Can you work these out from the model? Positions are in its coordinate system, mm. Give positions to 0.01 mm unless a question says otherwise; leave off trailing zeros. Loops run counter-clockwise (first coordinate to the right, second up) from the corner with the lowest first, then second, coordinate; pieces in that order, holes last. Notation, with made-up numbers: (70, 36.5) - (111, 36.5) arc R12 ccw to (111, 47.5) - close; hole circle Ø8 at (74, 37). An arc over 180 degrees is marked (long way). Answer in a Markdown table with one row per item.
Autodesk Inventor part; units mm, degrees
ref_plane "YZ Plane" through (0, 0, 0) normal (1, 0, 0) x (0, 1, 0)
ref_plane "XZ Plane" through (0, 0, 0) normal (0, 1, 0) x (-1, 0, 0)
ref_plane "XY Plane" through (0, 0, 0) normal (0, 0, 1) x (1, 0, 0)
sketch "Sketch1" plane through (0, 0, 0) normal (0, 1, 0) x (-1, 0, 0)
  circle A0 centre (0, 0) radius 12.7
  dimension "d0" = 25.4
extrude "Extrusion1" add sketch "Sketch1" along normal blind 5.8674
sketch "Sketch2" plane through (0, 5.8674, 0) normal (0, 1, 0) x (1, 0, 0)
  line L0 (0, 0) -> (-7.7692, 0)
  line L1 (-7.7692, 0) -> (-7.7692, 6.975)
  line L2 (-7.7692, 6.975) -> (0, 6.975)
  line L3 (0, 6.975) -> (0, 0)
extrude "Extrusion2" cut sketch "Sketch2" against normal blind 254
sketch "Sketch3" plane through (0, 5.8674, 0) normal (0, 1, 0) x (1, 0, 0)
  line L0 (0, 6.018) -> (5.0945, 6.018)
  line L1 (5.0945, 6.018) -> (5.0945, 4.5769)
  line L2 (5.0945, 4.5769) -> (0, 4.5769)
  line L3 (0, 4.5769) -> (0, 6.018)
  point P0 (0, 0)
extrude "Extrusion3" cut sketch "Sketch3" against normal blind 254
sketch "Sketch4" plane through (0, 5.8674, 0) normal (0, 1, 0) x (1, 0, 0)
  circle A0 centre (-2.0297, 0) radius 3.9608
  point P0 (0, 0)
extrude "Extrusion4" cut sketch "Sketch4" against normal blind 254
sketch "Sketch5" plane through (0, 5.8674, 0) normal (0, 1, 0) x (1, 0, 0)
  line L0 (12.2968, 4.5116) -> (-14.5211, 4.5116)
  line L1 (-14.5211, 4.5116) -> (-14.5211, 13.7027)
  line L2 (-14.5211, 13.7027) -> (12.2968, 13.7027)
  line L3 (12.2968, 13.7027) -> (12.2968, 4.5116)
  point P0 (0, 0)
extrude "Extrusion5" cut sketch "Sketch5" against normal blind 254
sketch "Sketch6" plane through (0, 5.8674, 0) normal (0, 1, 0) x (1, 0, 0)
  circle A0 centre (-3.4414, 4.0919) radius 9.7549
  point P0 (0, 0)
extrude "Extrusion6" cut sketch "Sketch6" against normal blind 254
properties part number "top hook"
Q1. For pin 1 (3 mm diameter, centred on x = 7.5, y = 4, fed in from +Z); pin 2 (2 mm diameter, centred on y = 5, z = -2, fed in from +X); pin 3 (2 mm diameter, centred on x = 2.5, y = 2.5, fed in from -Z), each with a flat end and sliding along its axis, tell me the tip position at first contact or that it passes through.
Checked values:
| item | result |
|---|---|
| pin 1 | stops at z = 11.19 |
| pin 2 | stops at x = 12.66 |
| pin 3 | stops at z = 2.76 |
Q2. If I drill on line 1 (X direction, y = 5.5, z = 4.75); line 2 (X direction, y = 4.6, z = 1.75); line 3 (Z direction, x = -3, y = 3.4), over which ranges is the centre line in solid material (lowest first)? Write a range as [from, to].
Checked values:
| item | result |
|---|---|
| line 1 | x = [-11.78, -7.56], [0.68, 11.78] |
| line 2 | x = [-12.58, -11.25], [4.37, 12.58] |
| line 3 | z = [5.65, 12.34] |
Q3. If we mould it in two halves opening along Y, with no side actions, what happens to faces 1 (the face through (3, 0, 6)), 2 (the face through (3, 5.867, 6)), 3 (the face through (-1.819, 2.975, 5.527))? For each: released by +Y, released by -Y, zero draft, split by the parting line, or undercut.
Checked values:
| item | result |
|---|---|
| face 1 | released by -Y |
| face 2 | released by +Y |
| face 3 | zero draft |
Q4. Imagine slicing it at A-A, the plane z = 0. Write out the boundary of the cut face in (x, y), and give its area (3 significant figures).
Checked values:
| item | result |
|---|---|
| outline | (-12.7, 0) - (-12.3, 0) - (-12.3, 5.87) - (-12.7, 5.87) - close; (5.41, 0) - (12.7, 0) - (12.7, 5.87) - (5.41, 5.87) - close |
| area | 45.1 mm² |
Q5. Imagine slicing it at B-B, the plane y = 4.35. Write out the boundary of the cut face in (x, z), and give its area (3 significant figures).
Checked values:
| item | result |
|---|---|
| outline | (-12.67, -0.92) arc R9.75 cw to (6.3, -4.51) - (11.87, -4.51) arc R12.7 ccw (long way) to start |
| area | 210 mm² |
Q6. Imagine slicing it at C-C, the plane z = 4.75. Write out the boundary of the cut face in (x, y).
Checked values:
| item | result |
|---|---|
| outline | (-11.78, 0) - (-7.56, 0) - (-7.56, 5.87) - (-11.78, 5.87) - close; (0.68, 0) - (11.78, 0) - (11.78, 5.87) - (0.68, 5.87) - close |
Q7. Imagine slicing it at D-D, the plane x = 0.5. Write out the boundary of the cut face in (y, z).
Checked values:
| item | result |
|---|---|
| outline | (0, 4.83) - (5.87, 4.83) - (5.87, 12.69) - (0, 12.69) - close |
